```python
from build123d import *

# Parameters (mm, degrees)
ESBO_O1_W                = 20
ESBO_O1_H                = 34
ESBO_O1_R                = 5
ESBO_O1_R_2              = 2.65
RESSALTO_EXTRUS_O1_DEPTH = 5
ESBO_O2_R                = 5
RESSALTO_EXTRUS_O2_DEPTH = 20
CORTE_EXTRUS_O1_START    = -9
CORTE_EXTRUS_O1_DEPTH    = 9
CORTE_EXTRUS_O3_REACH    = 46.227
ESBO_O5_R                = 1.65
CORTE_EXTRUS_O2_DEPTH    = 4
FILETE1_R                = 5
FILETE2_R                = 2
CORTE_EXTRUS_O4_START    = -15
ESBO_O6_R                = 4.75
CORTE_EXTRUS_O4_DEPTH    = 8
ESBO_O7_R                = 5
RESSALTO_EXTRUS_O3_DEPTH = 10
ESBO_O8_W                = 1
ESBO_O8_H                = 21.001730979
CORTE_EXTRUS_O5_DEPTH    = 7
ESBO_O10_R               = 4.5
CORTE_EXTRUS_O7_DEPTH    = 8
CHANFRO5_SIZE            = 1.732050808
CHANFRO5_SIZE_2          = 1
CORTE_EXTRUS_O8_START    = -10
CORTE_EXTRUS_O8_DEPTH    = 10
CHANFRO2_SIZE            = 0.5


with BuildPart() as part:
    # Esboço1 → Ressalto-extrusão1 (new body)
    with BuildSketch(Plane.XY):
        with Locations((10, 17)):
            Rectangle(ESBO_O1_W, ESBO_O1_H)
        with Locations((10, 17)):
            Circle(ESBO_O1_R, mode=Mode.SUBTRACT)
        with Locations((10, 29.5)):
            Circle(ESBO_O1_R_2, mode=Mode.SUBTRACT)
        with Locations((10, 4.5)):
            Circle(ESBO_O1_R_2, mode=Mode.SUBTRACT)
    extrude(amount=RESSALTO_EXTRUS_O1_DEPTH)

    # Esboço2 → Ressalto-extrusão2 (add)
    with BuildSketch(Plane(origin=(0, 0, 0), x_dir=(-1, 0, 0), z_dir=(0, 0, -1))):
        Polygon((0, 23.914879084), (-20, 28.90143914), (-20, 6.5), (0, 6.5), align=None)
        with Locations((-10, 17)):
            Circle(ESBO_O2_R, mode=Mode.SUBTRACT)
    extrude(amount=-RESSALTO_EXTRUS_O2_DEPTH)

    # Esboço3 → Corte-extrusão1 (cut)
    with BuildSketch(Plane.XY.offset(20).offset(CORTE_EXTRUS_O1_START)):
        with BuildLine():
            Line((6, 14), (6, 7.5))
            Line((6, 7.5), (0, 7.5))
            Line((0, 7.5), (0, 6.5))
            Line((0, 6.5), (7, 6.5))
            Line((7, 6.5), (7, 13))
            ThreePointArc((7, 13), (6.464466094, 13.464466094), (6, 14))
        make_face()
    extrude(amount=CORTE_EXTRUS_O1_DEPTH, mode=Mode.SUBTRACT)

    # Corte-extrusão3: up to this face of the body (flat: up to its plane)
    corte_extrus_o3_end = Plane(part.part.faces().sort_by_distance((20, 17.465309995, 9.140459531))[0])
    # Esboço5 → Corte-extrusão3 (cut, up to the picked face)
    with BuildSketch(Plane.ZY, mode=Mode.PRIVATE) as corte_extrus_o3_sk1:
        with Locations((16, 10)):
            Circle(ESBO_O5_R)
    corte_extrus_o3_tool1 = split(extrude(corte_extrus_o3_sk1.sketch, amount=-CORTE_EXTRUS_O3_REACH, mode=Mode.PRIVATE), bisect_by=corte_extrus_o3_end, keep=Keep.BOTH, mode=Mode.PRIVATE)
    add(corte_extrus_o3_tool1.solids().sort_by(Axis((0, 10, 16), (1, 0, 0)))[0], mode=Mode.SUBTRACT)

    # Esboço4 → Corte-extrusão2 (cut)
    with BuildSketch(Plane(origin=(20, 0, 0), x_dir=(0, 0, -1), z_dir=(1, 0, 0))):
        Polygon((-19.233161507, 10), (-17.616580754, 7.2), (-14.383419246, 7.2), (-12.766838493, 10), (-14.383419246, 12.8), (-17.616580754, 12.8), align=None)
    extrude(amount=-CORTE_EXTRUS_O2_DEPTH, mode=Mode.SUBTRACT)

    # Filete1
    filete1_edges = [part.edges().sort_by_distance(p)[0] for p in [
        (0, 23.914879084, 12.5),
        (20, 28.90143914, 12.5),
    ]]
    fillet(filete1_edges, radius=FILETE1_R)

    # Filete2
    filete2_edges = [part.edges().sort_by_distance(p)[0] for p in [
        (0, 34, 2.5),
        (20, 34, 2.5),
        (20, 0, 2.5),
        (0, 0, 2.5),
    ]]
    fillet(filete2_edges, radius=FILETE2_R)

    # Esboço6 → Corte-extrusão4 (cut)
    with BuildSketch(Plane.XY.offset(20).offset(CORTE_EXTRUS_O4_START)):
        with Locations((10, 4.5)):
            Circle(ESBO_O6_R)
    extrude(amount=CORTE_EXTRUS_O4_DEPTH, mode=Mode.SUBTRACT)

    # Esboço7 → Ressalto-extrusão3 (add)
    with BuildSketch(Plane(origin=(0, 0, 0), x_dir=(-1, 0, 0), z_dir=(0, 0, -1))):
        with Locations((-10, 17)):
            Circle(ESBO_O7_R)
    extrude(amount=-RESSALTO_EXTRUS_O3_DEPTH)

    # Esboço8 → Corte-extrusão5 (cut)
    with BuildSketch(Plane.ZY):
        with Locations((10.5, 17.00086549)):
            Rectangle(ESBO_O8_W, ESBO_O8_H)
    extrude(amount=-CORTE_EXTRUS_O5_DEPTH, mode=Mode.SUBTRACT)

    # Esboço10 → Corte-extrusão7 (cut)
    with BuildSketch(Plane.XY.offset(5)):
        with Locations((10, 29.5)):
            Circle(ESBO_O10_R)
    extrude(amount=CORTE_EXTRUS_O7_DEPTH, mode=Mode.SUBTRACT)

    # Chanfro5
    # the kernel refuses this chamfer: 1.732050808, 1 mm, written as the material it takes off along each edge
    with BuildSketch(Plane(origin=(18.789385955, 6.5, 13), x_dir=(0, 0.9998132206222079, -0.019326765612700685), z_dir=(-1, 0, 0))) as chanfro5_piece_1_section:
        Polygon((CHANFRO5_SIZE * 0.999813220373, -CHANFRO5_SIZE * 0.0193267656079), (-CHANFRO5_SIZE_2 * 0.0193267656127, -CHANFRO5_SIZE_2 * 0.999813220622), (0, 0), align=None)
    chanfro5_piece_1 = extrude(amount=16.270349926, mode=Mode.PRIVATE)
    chanfro5_piece_1 = chanfro5_piece_1 & Plane(origin=(10, 4.5, 13.142171605), x_dir=(1, 0, 0), z_dir=(0, 0, -1)) * Cylinder(4.75, 40, mode=Mode.PRIVATE)
    add(chanfro5_piece_1, mode=Mode.SUBTRACT)
    with BuildSketch(Plane(origin=(3.123434693, 24.693638818, 13), x_dir=(-0.014005792936040639, 0.056174167266921864, 0.9983227437537926), z_dir=(0.9702957262759956, 0.2419218955996716, 0))) as chanfro5_piece_2_section:
        Polygon((CHANFRO5_SIZE_2 * 0.998322743754, CHANFRO5_SIZE_2 * 0.0578938624027), (-CHANFRO5_SIZE * 0.0578938623883, CHANFRO5_SIZE * 0.998322743505), (0, 0), align=None)
    chanfro5_piece_2 = extrude(amount=10.993510061, mode=Mode.PRIVATE)
    chanfro5_piece_2 = chanfro5_piece_2 & Plane(origin=(10, 29.5, 13.381027624), x_dir=(1, 0, 0), z_dir=(0, 0, -1)) * Cylinder(4.5, 29, mode=Mode.PRIVATE)
    add(chanfro5_piece_2, mode=Mode.SUBTRACT)
    with BuildSketch(Plane(origin=(15, 22.501730979, 13), x_dir=(0.6367879492997914, 0.7710389793172368, 0), z_dir=(0.7710389793172368, -0.6367879492997914, 0))) as chanfro5_piece_3_section:
        Polygon((5 - CHANFRO5_SIZE, 0), (5, CHANFRO5_SIZE_2), (5, 0), align=None)
    chanfro5_piece_3 = revolve(axis=Axis((15, 22.501730979, 13), (0, 0, 1)), revolution_arc=53.552719823, mode=Mode.PRIVATE)
    chanfro5_piece_3 = chanfro5_piece_3 & Plane(origin=(10, 29.5, 13.480391977), x_dir=(1, 0, 0), z_dir=(0, 0, -1)) * Cylinder(4.5, 20, mode=Mode.PRIVATE)
    add(chanfro5_piece_3, mode=Mode.SUBTRACT)

    # Esboço11 → Corte-extrusão8 (cut)
    with BuildSketch(Plane.XY.offset(5).offset(CORTE_EXTRUS_O8_START)):
        with BuildLine():
            ThreePointArc((8.261466135, 6.5), (10, 1.85), (11.738533865, 6.5))
            ThreePointArc((11.738533865, 6.5), (10, 7.15), (8.261466135, 6.5))
        make_face()
    extrude(amount=CORTE_EXTRUS_O8_DEPTH, mode=Mode.SUBTRACT)

    # Chanfro2
    chanfro2_edges = [part.edges().sort_by_distance(p)[0] for p in [
        (10, 34, 0),
        (20, 17, 0),
        (10, 0, 0),
        (0, 17, 0),
        (0.585786438, 33.414213562, 0),
        (0.585786438, 0.585786438, 0),
        (19.414213562, 0.585786438, 0),
        (19.414213562, 33.414213562, 0),
        (7.35, 29.5, 0),
        (8.261466135, 2.5, 0),
        (13.535533906, 20.535533906, 20),
    ]]
    chamfer(chanfro2_edges, length=CHANFRO2_SIZE)


solid = part.part
```
The listing builds one solid part. Answer for the finished solid, in the listing's coordinates (mm). A direction names the side the tool comes from. Give positions to 0.01 mm unless a question says otherwise; leave off trailing zeros. Loops run counter-clockwise (first coordinate to the right, second up) from the corner with the lowest first, then second, coordinate; pieces in that order, holes last. Notation, with made-up numbers: M 0,61.25 L 43,61.25 A35 ccw 43,95.25 Z; hole C 3,32.25 d2. An arc over 180 degrees is marked long. One line per item, written item: value.
1. Each of these flat-tipped pins is pushed along its axis until it touches: P1, Ø5, axis at x = 10, y = 4.5, coming from the -Z side; P2, Ø2.5, axis at x = 2.5, z = 7, coming from the -Y side; P3, Ø0.5, axis at y = 23, z = 10.5, coming from the -X side. Where does it stop, or does it pass through?
Found:
P1: z = 13.71
P2: y = 6.5
P3: x = 7
2. For faces 5 (the face through (13, 21, 15)), 6 (the face through (10.73, 26, 13.67)), 7 (the face through (7.609, 25.812, 15.728)), 8 (the face through (15, 6.5, 14)), 9 (the face through (18, 12.8, 16)), determine the directions among +Z, -Z, +X, -X, +Y, -Y from which every point of the face is accessible in a straight line to the end or side of a thin tool.
Found:
face 5: +Z
face 6: +Y
face 7: +Z, -X, +Y
face 8: +Z, +X, -X, -Y
face 9: +X
3. Section D-D on z = 16 is taken. Determine the outline of the cut face in (x, y).
Found:
outline: M 0,7.5 L 6,7.5 L 6,8.35 L 0,8.35 Z; M 0,11.65 L 6,11.65 L 6,14 A5 cw long 7,13 L 7,11.65 L 16,11.65 L 16,12.8 L 20,12.8 L 20,22.5 A5 ccw 13.79,27.35 L 3.79,24.86 A5 ccw 0,20.01 Z; M 7,6.5 L 20,6.5 L 20,7.2 L 16,7.2 L 16,8.35 L 7,8.35 Z
4. For a pull along X with two mould halves and no side action, classify faces 1 (the face through (11.437, 9.368, 17.524)), 2 (the face through (19.15, 33.17, 0.14)), 3 (the face through (7, 10, 14)), 4 (the face through (10.71, 7.38, 13.49)) as pulls with the +X half, pulls with the -X half, needs draft (parallel to the pull), parting line crosses it, or undercut.
Found:
face 1: needs draft
face 2: pulls with the +X half
face 3: undercut
face 4: undercut
5. Section B-B on x = 10 is taken. State how many separate pieces and enclosed holes the cut face has, plus the area to 3 significant figures.
Found:
separate pieces: 3
enclosed holes: 1
area: 271 mm^2
6. Section C-C on y = 17 is taken. Determine the outline of the cut face in (x, z).
Found:
outline: M 0,0.5 L 0.5,0 L 19.5,0 L 20,0.5 L 20,20 L 15.5,20 L 15,19.5 L 15,10 L 0,10 Z; M 0,11 L 5,11 L 5,19.5 L 4.5,20 L 0,20 Z
7. Find the intervals of material crossed by probe 1 along X at (y, z) = (20, 18.75); probe 2 along X at (y, z) = (17, 12.5); probe 3 along Z at (x, y) = (2.5, 8), in increasing order.
Found:
probe 1: 0 to 6, 14 to 20
probe 2: 0 to 5, 15 to 20
probe 3: 0 to 10, 11 to 20
8. Section A-A on z = 4 is taken. Determine the outline of the cut face in (x, y).
Found:
outline: M 0,2 A2 ccw 2,0 L 18,0 A2 ccw 20,2 L 20,32 A2 ccw 18,34 L 2,34 A2 ccw 0,32 Z; hole C 10,4.5 d5.3; hole C 10,29.5 d5.3
